The listing builds one solid part. Answer for the finished solid, in the listing's coordinates (mm). Face numbers are marked on the shaded views. A direction names the side the tool comes from. Give positions to 0.01 mm unless a question says otherwise; leave off trailing zeros. Order: outer loops, then holes, each group sorted by start corner. A loop starts at its lowest first (then second) coordinate and runs counter-clockwise, first axis right, second up. Notation, with made-up numbers: (7, -19) -> (35, -19) arc R13 cw to (35, -10) -> close; hole circle Ø10 at (7.25, -4.5). An arc over 180 degrees is marked (long way). Answer as a JSON object with one key per item and string values. Group by question number.
```python
from build123d import *

# Parameters (mm, degrees)
SKETCH001_W     = 84
SKETCH001_H     = 44
SKETCH001_W_2   = 80.8
SKETCH001_H_2   = 40.8
PAD_DEPTH       = 20.6
SKETCH002_W     = 84
SKETCH002_H     = 44
PAD001_DEPTH    = 2
SKETCH003_R     = 3
SKETCH003_R_2   = 1.55
PAD002_DEPTH    = 4.4
SKETCH004_W     = 8.5
SKETCH004_H     = 3.45
POCKET_DEPTH    = 1.6
CHAMFER_SIZE    = 0.8
CHAMFER001_SIZE = 0.4
FILLET_R        = 1
CHAMFER002_SIZE = 0.4


with BuildPart() as part:
    # Sketch001 → Pad (new body)
    with BuildSketch(Plane.XY):
        with Locations((42, 22)):
            Rectangle(SKETCH001_W, SKETCH001_H)
        with Locations((42, 22)):
            Rectangle(SKETCH001_W_2, SKETCH001_H_2, mode=Mode.SUBTRACT)
    extrude(amount=PAD_DEPTH)

    # Sketch002 (on Face9 of Pad) → Pad001 (join)
    with BuildSketch(Plane(origin=(0, 0, 0), x_dir=(1, 0, 0), z_dir=(0, 0, -1))):
        with Locations((42, -22)):
            Rectangle(SKETCH002_W, SKETCH002_H)
    extrude(amount=PAD001_DEPTH)

    # Sketch003 (on Face8 of Pad001) → Pad002 (join)
    with BuildSketch(Plane.XY):
        with Locations((6, 38)):
            Circle(SKETCH003_R)
        with Locations((6, 38)):
            Circle(SKETCH003_R_2, mode=Mode.SUBTRACT)
        with Locations((78, 38)):
            Circle(SKETCH003_R)
        with Locations((78, 38)):
            Circle(SKETCH003_R_2, mode=Mode.SUBTRACT)
        with Locations((78, 6)):
            Circle(SKETCH003_R)
        with Locations((78, 6)):
            Circle(SKETCH003_R_2, mode=Mode.SUBTRACT)
        with Locations((6, 6)):
            Circle(SKETCH003_R)
        with Locations((6, 6)):
            Circle(SKETCH003_R_2, mode=Mode.SUBTRACT)
    extrude(amount=PAD002_DEPTH)

    # Sketch004 (on Face4 of Pad002) → Pocket (cut)
    with BuildSketch(Plane.YZ.offset(84)):
        with Locations((22, 2.175)):
            Rectangle(SKETCH004_W, SKETCH004_H)
    extrude(amount=-POCKET_DEPTH, mode=Mode.SUBTRACT)

    # Chamfer
    chamfer_edges = [part.edges().sort_by_distance(p)[0] for p in [
        (1.6, 22, 20.6),
        (42, 42.4, 20.6),
        (82.4, 22, 20.6),
        (42, 1.6, 20.6),
    ]]
    chamfer(chamfer_edges, length=CHAMFER_SIZE)

    # Chamfer001
    chamfer001_edges = [part.edges().sort_by_distance(p)[0] for p in [
        (4.45, 38, 4.4),
        (76.45, 38, 4.4),
        (76.45, 6, 4.4),
        (4.45, 6, 4.4),
    ]]
    chamfer(chamfer001_edges, length=CHAMFER001_SIZE)

    # Fillet
    fillet_edges = [part.edges().sort_by_distance(p)[0] for p in [
        (0, 0, 9.3),
        (84, 0, 9.3),
        (84, 44, 9.3),
        (0, 44, 9.3),
    ]]
    fillet(fillet_edges, radius=FILLET_R)

    # Chamfer002
    chamfer002_edges = [part.edges().sort_by_distance(p)[0] for p in [
        (84, 22, 3.9),
        (84, 26.25, 2.175),
        (84, 22, 0.45),
        (84, 17.75, 2.175),
    ]]
    chamfer(chamfer002_edges, length=CHAMFER002_SIZE)


solid = part.part
```
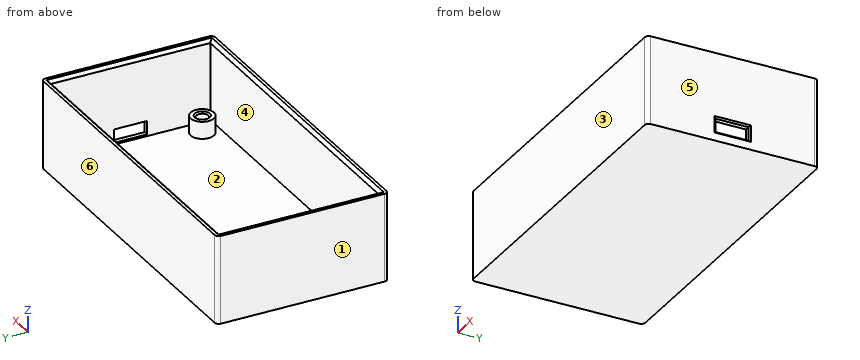
(1) A cutting plane is placed at A-A (y = 21). Determine the outline of the cut face in (x, z), and give its area (3 significant figures).
(2) Which of the six approach directions +Z, -Z, +X, -X, +Y, -Y give full straight-line access (tool end or side, diameter ignored) to the marked faces 1 and 2?
(3) Flat-ended cylindrical pins translate along their axes: pin 1 Ø0.9 at (x, y) = (78, 5.5) entering from +Z; pin 2 Ø3.5 at (x, y) = (6.5, 38.5) entering from +Z. Find the tip coordinate at first contact, or state that the pin passes through.
(4) A cutting plane is placed at B-B (z = 8.75). Determine the outline of the cut face in (x, y), and give its area (3 significant figures).
(5) Find the intervals of material crossed by line 1 along Y through (x, z) = (78, 3.1); line 2 along Y through (x, z) = (60.5, 16); line 3 along X through (y, z) = (26.5, 7.25), in increasing order. Write a range as [from, to].
(6) For a pull along Y with two mould halves and no side action, classify the marked faces 3, 4, 5 and 6 as +Y half, -Y half, draft (parallel to the pull), parting line (faces both ways), or undercut.
Check sheet entries:
{
 "1": {"outline": "(0, -2) -> (84, -2) -> (84, 0.05) -> (83.6, 0.45) -> (82.4, 0.45) -> (82.4, 0) -> (1.6, 0) -> (1.6, 19.8) -> (0.8, 20.6) -> (0, 20.6) -> close; (82.4, 3.9) -> (83.6, 3.9) -> (84, 4.3) -> (84, 20.6) -> (83.2, 20.6) -> (82.4, 19.8) -> close", "area": "228 mm2"},
 "2": {"face 1": "+Z, -Z, -X, +Y, -Y", "face 2": "+Z"},
 "3": {"pin 1": "stops at z = 0", "pin 2": "stops at z = 4.4"},
 "4": {"outline": "(0, 1) arc R1 ccw to (1, 0) -> (83, 0) arc R1 ccw to (84, 1) -> (84, 43) arc R1 ccw to (83, 44) -> (1, 44) arc R1 ccw to (0, 43) -> close; hole (1.6, 1.6) -> (82.4, 1.6) -> (82.4, 42.4) -> (1.6, 42.4) -> close", "area": "399 mm2"},
 "5": {"line 1": "y = [0, 1.6], [3, 4.45], [7.55, 9], [35, 36.45], [39.55, 41], [42.4, 44]", "line 2": "y = [0, 1.6], [42.4, 44]", "line 3": "x = [0, 1.6], [82.4, 84]"},
 "6": {"face 3": "-Y half", "face 4": "undercut", "face 5": "draft", "face 6": "+Y half"}
}
